from build123d import *

# Parameters (mm, degrees)
BOX_W               = 20
BOX_H               = 10
BOX_DEPTH           = 10
BOX_PLACEMENT_ANGLE = 14
ARRAY_COUNT         = 8
CYLINDER001_R       = 20
CYLINDER001_DEPTH   = 20
CYLINDER_R          = 30
CYLINDER_DEPTH      = 100


with BuildPart() as obj1:
    # Box → Box (new body)
    with BuildSketch(Plane.XY):
        with Locations((10, 5)):
            Rectangle(BOX_W, BOX_H)
    extrude(amount=BOX_DEPTH)


with BuildPart() as obj1_1:
    # Box placement: moved
    add(obj1.part.moved(Location((15, 0, 90))).rotate(Axis((15, 0, 90), (0, 0, 1)), BOX_PLACEMENT_ANGLE))

    # Array: obj1 ×8 about axis
    array_axis = Axis((0, 0, 1), (0, 0, 1))


with BuildPart() as obj1_2:
    add(obj1_1.part)
    for i in range(1, ARRAY_COUNT):
        add(obj1_1.part.rotate(array_axis, i * 360 / ARRAY_COUNT))


with BuildPart() as cylinder001:
    # Cylinder001 → Cylinder001 (new body)
    with BuildSketch(Plane.XY.offset(80)):
        Circle(CYLINDER001_R)
    extrude(amount=CYLINDER001_DEPTH)


with BuildPart() as torre:
    # Cylinder → Cylinder (new body)
    with BuildSketch(Plane.XY):
        Circle(CYLINDER_R)
    extrude(amount=CYLINDER_DEPTH)

    # Cut: cut Cylinder001
    add(cylinder001.part, mode=Mode.SUBTRACT)

    # Cut001: cut obj1
    add(obj1_2.part, mode=Mode.SUBTRACT)


solid = torre.part
Here's how the part is built. I have some questions about the finished solid (model axes, mm). A direction names the side the tool comes from. Give positions to 0.01 mm unless a question says otherwise; leave off trailing zeros. Order: outer loops, then holes, each group sorted by start corner. A loop starts at its lowest first (then second) coordinate and runs counter-clockwise, first axis right, second up. Notation, with made-up numbers: (-36, 41.5) -> (6, 41.5) arc R20 ccw to (6, 51.5) -> close; hole circle Ø2 at (68.5, 82.25). An arc over 180 degrees is marked (long way). Use a Markdown table: item, result. Add a question column.
Item 1: Will these pins go through, and if not, where does the flat tip stop? pin 1 (3 mm diameter, centred on y = 13.5, z = 53, fed in from -X); pin 2 (4 mm diameter, centred on x = 22, y = -11, fed in from +Z); pin 3 (3 mm diameter, centred on y = -3.5, z = 17.5, fed in from -X).
Item 2: I need wall thicknesses on line 1 (Y direction, x = 0, z = 85); line 2 (Y direction, x = 3.5, z = 29.5). Which ranges of each line are inside material? Lowest first, please.
Item 3: Imagine slicing it at B-B on y = 0. Please give me the cut outline in (x, z), plus the area to 3 significant figures.
Item 4: For faces 4 (the face through (-24.799, -2.443, 94.93)), 5 (the face through (6.933, 23.909, 94.93)), 6 (the face through (-12, 21.8, 94.9)), 7 (the face through (-19.263, 15.808, 94.93)), 8 (the face through (0, 0, 0)), which set-ups out of +Z, -Z, +X, -X, +Y, -Y let a thin tool reach every point of the face, with its end or its side?
Item 5: Imagine slicing it at D-D on x = 7. Please give me the cut outline in (y, z) (3 decimals).
Item 6: If we mould it in two halves opening along Y, with no side actions, what happens to faces 1 (the face through (-16, 20, 100)), 2 (the face through (-15.808, -19.263, 94.93)), 3 (the face through (-19.98, 0.88, 87.64))? For each: pulls with the +Y half, pulls with the -Y half, needs draft (parallel to the pull), parting line crosses it, or undercut.
Item 7: Imagine slicing it at A-A on z = 93. Give the number of separate pieces and of enclosed holes in the cut face, plus the area to 3 significant figures.
Data:
| question | item | result |
|---|---|---|
| 1 | pin 1 | stops at x = -27.5 |
| 1 | pin 2 | stops at z = 90 |
| 1 | pin 3 | stops at x = -29.93 |
| 2 | line 1 | y = -30 to -20, 20 to 30 |
| 2 | line 2 | y = -29.8 to 29.8 |
| 3 | outline | (-30, 0) -> (30, 0) -> (30, 100) -> (20, 100) -> (20, 80) -> (-20, 80) -> (-20, 100) -> (-30, 100) -> close |
| 3 | area | 5,200 mm² |
| 4 | face 4 | +Z |
| 4 | face 5 | +Z, -Y |
| 4 | face 6 | +Z, +Y |
| 4 | face 7 | +Z, -X |
| 4 | face 8 | -Z, +X, -X, +Y, -Y |
| 5 | outline | (-29.172, 0) -> (29.172, 0) -> (29.172, 100) -> (24.02, 100) -> (24.02, 90) -> (18.735, 90) -> (18.735, 80) -> (-18.735, 80) -> (-18.735, 90) -> (-29.172, 90) -> close |
| 6 | face 1 | needs draft |
| 6 | face 2 | pulls with the -Y half |
| 6 | face 3 | undercut |
| 7 | separate pieces | 8 |
| 7 | enclosed holes | 0 |
| 7 | area | 764 mm² |
